from build123d import *

# Parameters (mm, degrees)
F0_R     = 3.1877
F1_DEPTH = 25.4
F3_DEPTH = 3.175
F4_SIZE  = 1.6002
F5_R     = 4.7625
F6_DEPTH = 19.05


with BuildPart() as f1:
    # F0 (on Top) → F1 (new body)
    with BuildSketch(Plane.XY):
        with BuildLine():
            Line((-12.7, 50.8), (-50.8, 50.8))
            Line((-50.8, 50.8), (-50.8, -50.8))
            Line((-50.8, -50.8), (-9.525, -50.8))
            Line((-9.525, -50.8), (-9.525, -23.0124))
            ThreePointArc((-9.525, -23.0124), (0, -13.4874), (9.525, -23.0124))
            Line((9.525, -23.0124), (9.525, -50.8))
            Line((9.525, -50.8), (50.8, -50.8))
            Line((50.8, -50.8), (50.8, 50.8))
            Line((50.8, 50.8), (12.7, 50.8))
            Line((12.7, 50.8), (12.7, 25.4))
            Line((12.7, 25.4), (-12.7, 25.4))
            Line((-12.7, 25.4), (-12.7, 50.8))
        make_face()
        with Locations((0, -7.1374)):
            Circle(F0_R, mode=Mode.SUBTRACT)
    extrude(amount=F1_DEPTH)

    # F2 (on face) → F3 (cut)
    with BuildSketch(Plane(origin=(0, 0, 0), x_dir=(1, 0, 0), z_dir=(0, 0, -1))):
        with BuildLine():
            Line((-12.7, -22.225), (-12.7, -25.4))
            Line((-12.7, -25.4), (12.7, -25.4))
            Line((12.7, -25.4), (12.7, -22.225))
            ThreePointArc((12.7, -22.225), (9.525, -19.05), (6.35, -22.225))
            Line((6.35, -22.225), (-6.35, -22.225))
            ThreePointArc((-6.35, -22.225), (-9.525, -19.05), (-12.7, -22.225))
        make_face()
    extrude(amount=-F3_DEPTH, mode=Mode.SUBTRACT)

    # F4
    f4_edges = [f1.edges().sort_by_distance(p)[0] for p in [
        (-50.8, 0, 25.4),
        (-30.1625, -50.8, 25.4),
        (30.1625, -50.8, 25.4),
        (50.8, 0, 25.4),
        (31.75, 50.8, 25.4),
        (-31.75, 50.8, 25.4),
    ]]
    chamfer(f4_edges, length=F4_SIZE)

    # F5 (on face) → F6 (cut)
    with BuildSketch(Plane(origin=(0, 25.4, 0), x_dir=(-1, 0, 0), z_dir=(0, 1, 0))):
        with Locations((0, 14.3002)):
            Circle(F5_R)
    extrude(amount=-F6_DEPTH, mode=Mode.SUBTRACT)


solid = f1.part
Input: part model. Units: mm. Frame: model coordinates. A direction names the side the tool comes from. Give positions to 0.01 mm unless a question says otherwise; leave off trailing zeros. Order: outer loops, then holes, each group sorted by start corner. A loop starts at its lowest first (then second) coordinate and runs counter-clockwise, first axis right, second up. Notation, with made-up numbers: (-1.75, -24) -> (45.25, -24) arc R4 ccw to (45.25, -18) -> close; hole circle Ø8 at (27, -20). An arc over 180 degrees is marked (long way). Use one line per item in the form item = value.
1) Section A-A, the plane x = 0. Return loops of the section in (y, z) (3 decimals).
Response values:
outline = (-13.487, 0) -> (-10.325, 0) -> (-10.325, 25.4) -> (-13.487, 25.4) -> close; (-3.95, 0) -> (22.225, 0) -> (22.225, 3.175) -> (25.4, 3.175) -> (25.4, 9.538) -> (6.35, 9.538) -> (6.35, 19.063) -> (25.4, 19.063) -> (25.4, 25.4) -> (-3.95, 25.4) -> close
2) Section C-C, the plane z = 12. Return loops of the section in (x, y) (3 decimals), and give its area (3 significant figures).
Response values:
outline = (-50.8, -50.8) -> (-9.525, -50.8) -> (-9.525, -23.012) arc R9.525 cw to (9.525, -23.012) -> (9.525, -50.8) -> (50.8, -50.8) -> (50.8, 50.8) -> (12.7, 50.8) -> (12.7, 25.4) -> (4.17, 25.4) -> (4.17, 6.35) -> (-4.17, 6.35) -> (-4.17, 25.4) -> (-12.7, 25.4) -> (-12.7, 50.8) -> (-50.8, 50.8) -> close; hole circle Ø6.375 at (0, -7.137)
area = 8,810 mm^2
3) Reachability of faces 4 (the cylindrical face through (1.03, 16.01, 9.65)), 5 (the flat face through (-9.525, -37, 13)), 6 (the flat face through (0, 25.4, 9)), 7 (the flat face through (0, 23, 3.175)) from +Z, -Z, +X, -X, +Y, -Y: full face, straight path, thin tool, end or side. Return the list, or none.
Response values:
face_4 = +Y
face_5 = +Z, -Z, -Y
face_6 = +Z, -Z, +Y
face_7 = -Z, +Y
4) First-contact query: pin 1 Ø1.9 at (x, y) = (2, 23.5) entering from -Z (3 decimals); pin 2 Ø3.5 at (x, z) = (2.5, 2) entering from +Y; pin 3 Ø8.5 at (x, z) = (0, 14.3) entering from +Y. Flat tips, straight axial feed; report the tip coordinate or a pass-through.
Response values:
pin_1 = 3.175
pin_2 = 25.4
pin_3 = 6.35
5) Section D-D, the plane z = 5.5. Return loops of the section in (x, y) (3 decimals).
Response values:
outline = (-50.8, -50.8) -> (-9.525, -50.8) -> (-9.525, -23.012) arc R9.525 cw to (9.525, -23.012) -> (9.525, -50.8) -> (50.8, -50.8) -> (50.8, 50.8) -> (12.7, 50.8) -> (12.7, 25.4) -> (-12.7, 25.4) -> (-12.7, 50.8) -> (-50.8, 50.8) -> close; hole circle Ø6.375 at (0, -7.137)
6) Mould query, pull axis Y, two halves, no side actions, for faces 1 (the cylindrical face through (-0.69, -10.25, 12.52)), 2 (the flat face through (0, 6.35, 14)), 3 (the flat face through (30, -50.8, 12)). Classes: pulls with the +Y half, pulls with the -Y half, needs draft (parallel to the pull), parting line crosses it, or undercut.
Response values:
face_1 = undercut
face_2 = pulls with the +Y half
face_3 = pulls with the -Y half
7) Line query: probe 1 along Y at (x, z) = (0, 5.75); probe 2 along X at (y, z) = (45.5, 20.25); probe 3 along Y at (x, z) = (0, 16.25). Output: solid intervals per line, ascending.
Response values:
probe_1 = -13.49 to -10.33, -3.95 to 25.4
probe_2 = -50.8 to -12.7, 12.7 to 50.8
probe_3 = -13.49 to -10.33, -3.95 to 6.35
8) Section B-B, the plane y = 39. Return loops of the section in (x, z), and give its area (3 significant figures).
Response values:
outline = (-50.8, 0) -> (-12.7, 0) -> (-12.7, 25.4) -> (-49.2, 25.4) -> (-50.8, 23.8) -> close; (12.7, 0) -> (50.8, 0) -> (50.8, 23.8) -> (49.2, 25.4) -> (12.7, 25.4) -> close
area = 1,930 mm^2
